from build123d import *

# Parameters (mm, degrees)
SKETCH1_R               = 86.36
SKETCH1_R_2             = 83.185
BOSS_EXTRUDE1_DEPTH     = 25.4
SKETCH2_R               = 3.175
CUT_EXTRUDE1_DEPTH      = 87.36
CUT_EXTRUDE1_DEPTH_BACK = 87.36
SKETCH3_R               = 2.3368
CUT_EXTRUDE2_DEPTH      = 87.3600001
CUT_EXTRUDE2_DEPTH_BACK = 87.3600001


with BuildPart() as part:
    # Sketch1 → Boss-Extrude1 (new body)
    with BuildSketch(Plane(origin=(0, 0, 0), x_dir=(1, 0, 0), z_dir=(0, 1, 0))):
        Circle(SKETCH1_R)
        Circle(SKETCH1_R_2, mode=Mode.SUBTRACT)
    extrude(amount=BOSS_EXTRUDE1_DEPTH)

    # Sketch2 → Cut-Extrude1 (cut, two sides)
    with BuildSketch(Plane(origin=(0, 0, 0), x_dir=(0, 0, -1), z_dir=(1, 0, 0))) as cut_extrude1_sk:
        with Locations((0, 12.7)):
            Circle(SKETCH2_R)
    extrude(amount=CUT_EXTRUDE1_DEPTH, mode=Mode.SUBTRACT)
    extrude(cut_extrude1_sk.sketch, amount=-CUT_EXTRUDE1_DEPTH_BACK, mode=Mode.SUBTRACT)

    # Sketch3 → Cut-Extrude2 (cut, two sides)
    with BuildSketch(Plane.XY) as cut_extrude2_sk:
        with Locations((0, 12.7)):
            Circle(SKETCH3_R)
    extrude(amount=CUT_EXTRUDE2_DEPTH, mode=Mode.SUBTRACT)
    extrude(cut_extrude2_sk.sketch, amount=-CUT_EXTRUDE2_DEPTH_BACK, mode=Mode.SUBTRACT)


solid = part.part
Design review of the part built by this model. Coordinates are the model's own, in mm. Give positions to 0.01 mm unless a question says otherwise; leave off trailing zeros. Loops run counter-clockwise (first coordinate to the right, second up) from the corner with the lowest first, then second, coordinate; pieces in that order, holes last. Notation, with made-up numbers: M -5.75,74.5 L 53.25,74.5 A28 ccw 53.25,108.5 Z; hole C 81,79.25 d5. An arc over 180 degrees is marked long. One line per question, with ' | ' between items. Start each with the question number.
1. To check wall thickness, follow L1, parallel to Y at x = 84.2, z = 0 (3 decimals); L2, parallel to X at y = 19.75, z = 0 (3 decimals); L3, parallel to Y at x = 0, z = 84.4. State the ranges of each line that lie inside material, in increasing order.
2. Add section C-C (y = 12.7). Write out the cut boundary in (x, z) (3 decimals).
3. The part is to be moulded in two halves that separate along Z. For faces 1 (the face through (84.7, 9.9, -1.5)), 2 (the face through (-0.51, 10.42, 84.73)), 3 (the face through (-63.65, 12.52, -58.37)), say which applies: released by +Z, released by -Z, zero draft, split by the parting line, or undercut.
4. Insertion check: P1, Ø4, axis at x = -47, y = 22, coming from the -Z side; P2, Ø7.5, axis at x = 0, y = 12.7, coming from the +Z side; P3, Ø10, axis at x = 51, y = 18.5, coming from the +Z side; P4, Ø1.5, axis at x = -33, y = 10, coming from the -Z side. Each pin has a flat end and moves straight along its axis. Give the tip position at first contact, or say it passes through.
5. Add section A-A (z = 0). Write out the cut boundary in (x, y) (3 decimals), plus the area to 3 significant figures.
6. Add section D-D (z = 33.5). Write out the cut boundary in (x, y), plus the area to 3 significant figures.
7. Add section B-B (x = -50.5). Write out the cut boundary in (y, z), plus the area to 3 significant figures.
Worked out:
1) L1: y = 0 to 9.525, 15.875 to 25.4 | L2: x = -86.36 to -83.185, 83.185 to 86.36 | L3: y = 0 to 10.36, 15.04 to 25.4
2) outline: M -86.302,-3.175 A86.36 ccw -2.337,-86.328 L -2.337,-83.152 A83.185 cw -83.124,-3.175 Z; M -86.302,3.175 L -83.124,3.175 A83.185 cw -2.337,83.152 L -2.337,86.328 A86.36 ccw Z; M 2.337,-86.328 A86.36 ccw 86.302,-3.175 L 83.124,-3.175 A83.185 cw 2.337,-83.152 Z; M 2.337,83.152 A83.185 cw 83.124,3.175 L 86.302,3.175 A86.36 ccw 2.337,86.328 Z
3) face 1: undercut | face 2: zero draft | face 3: split by the parting line
4) P1: stops at z = -73.71 | P2: stops at z = 86.36 | P3: stops at z = 73.09 | P4: stops at z = -80.11
5) outline: M -86.36,0 L -83.185,0 L -83.185,9.525 L -86.36,9.525 Z; M -86.36,15.875 L -83.185,15.875 L -83.185,25.4 L -86.36,25.4 Z; M 83.185,0 L 86.36,0 L 86.36,9.525 L 83.185,9.525 Z; M 83.185,15.875 L 86.36,15.875 L 86.36,25.4 L 83.185,25.4 Z | area: 121 mm²
6) outline: M -79.6,0 L -76.14,0 L -76.14,25.4 L -79.6,25.4 Z; M 76.14,0 L 79.6,0 L 79.6,25.4 L 76.14,25.4 Z | area: 176 mm²
7) outline: M 0,-70.06 L 25.4,-70.06 L 25.4,-66.1 L 0,-66.1 Z; M 0,66.1 L 25.4,66.1 L 25.4,70.06 L 0,70.06 Z | area: 201 mm²
